Work out the finished part from the listing and answer in its coordinate system (mm). A direction names the side the tool comes from. Round coordinates to 2 decimals unless told otherwise and drop trailing zeros. Write each loop counter-clockwise with the first axis right and the second up, starting at its lowest first coordinate (ties: lowest second). Pieces come first, ordered by that corner, then holes. Notation, with made-up numbers: M 82,74.5 L 126,74.5 A15 ccw 126,93.5 Z; hole C 80,-38 d3. An arc over 180 degrees is marked long. One line per item, written item: value. Start each with the question number.
Q1. Find section C-C (y = 9). Write down the section's boundary in (x, z).
Q2. Find section B-B (z = 3). Write down the section's boundary in (x, y).
Q3. Consider probe 1 along Y at (x, z) = (-27, 1.5); probe 2 along X at (y, z) = (3.5, 1.5); probe 3 along Z at (x, y) = (-9.5, -13). Determine where each line is inside the solid, lowest interval first.
Q4. Given pin 1 Ø1 at (y, z) = (-20.5, 2.5) entering from -X; pin 2 Ø2 at (y, z) = (-31, 2.5) entering from -X; pin 3 Ø1 at (x, z) = (-12.5, 1) entering from +Y, each flat-ended and moving along its own axis, determine where each tip first touches the part or whether it passes through.
Q5. A tool of negligible diameter and unlimited length cuts with its end or side. For faces 4 (the cylindrical face through (4.336, -19.524, 2.465)), 5 (the cylindrical face through (-6.335, 4.375, 6.972)), from which of +Z, -Z, +X, -X, +Y, -Y can it reach the whole face along a straight path? Write none if from no direction.
Q6. Find section A-A (y = 0). Write down the section's boundary in (x, z).
Q7. Find section D-D (z = 7.75). Count the separate pieces of the cut face and the enclosed holes in it, and give its area (3 significant figures).
Q8. The mould has two halves that part along X. Classify faces 1 (the cylindrical face through (-29.11, 26.7, 4.44)), 2 (the flat face through (8, 1, 9)), 3 (the flat face through (-4, 0, 5)): released by +X, released by -X, zero draft, split by the parting line, or undercut.
from build123d import *

# Parameters (mm, degrees)
SKETCH_1_R          = 39.5
EXTRUDE_1_DEPTH     = 9
SKETCH_2_R          = 20
CUT_EXTRUDE_1_DEPTH = 5
SKETCH_3_R          = 1.5
CUT_EXTRUDE_2_DEPTH = 57.581799194
SKETCH_4_R          = 1.5
CUT_EXTRUDE_3_DEPTH = 57.084757288


with BuildPart() as part:
    # 草图1 → 凸台-拉伸1 (new body)
    with BuildSketch(Plane.XY):
        Circle(SKETCH_1_R)
    extrude(amount=EXTRUDE_1_DEPTH)

    # 草图2 → 切除-拉伸1 (cut)
    with BuildSketch(Plane(origin=(0, 0, 0), x_dir=(-1, 0, 0), z_dir=(0, 0, -1))):
        Circle(SKETCH_2_R)
    extrude(amount=-CUT_EXTRUDE_1_DEPTH, mode=Mode.SUBTRACT)

    # 草图3 → 切除-拉伸2 (cut, through all)
    with BuildSketch(Plane(origin=(0, 0, 0), x_dir=(-1, 0, 0), z_dir=(0, 0, -1))):
        with Locations((1.136716128, -32.98041656)):
            Circle(SKETCH_3_R)
        with Locations((-29.130236632, 15.505783236)):
            Circle(SKETCH_3_R)
        with Locations((27.993520504, 17.474633324)):
            Circle(SKETCH_3_R)
    extrude(amount=-CUT_EXTRUDE_2_DEPTH, mode=Mode.SUBTRACT)

    # 草图4 → 切除-拉伸3 (cut, through all)
    with BuildSketch(Plane(origin=(0, 0, 5), x_dir=(-1, 0, 0), z_dir=(0, 0, -1))):
        Circle(SKETCH_4_R)
        with Locations((-4.949747468, 4.949747468)):
            Circle(SKETCH_4_R)
        with Locations((4.949747468, 4.949747468)):
            Circle(SKETCH_4_R)
        with Locations((4.949747468, -4.949747468)):
            Circle(SKETCH_4_R)
        with Locations((-4.949747468, -4.949747468)):
            Circle(SKETCH_4_R)
    extrude(amount=-CUT_EXTRUDE_3_DEPTH, mode=Mode.SUBTRACT)


solid = part.part
The answers:
1. outline: M -38.46,0 L -17.86,0 L -17.86,5 L 17.86,5 L 17.86,0 L 38.46,0 L 38.46,9 L -38.46,9 Z
2. outline: C 0,0 d79; hole C -27.99,17.47 d3; hole C 0,0 d40; hole C -1.14,-32.98 d3; hole C 29.13,15.51 d3
3. probe 1: -28.83 to 16.35, 18.6 to 28.83
3. probe 2: -39.34 to -19.69, 19.69 to 39.34
3. probe 3: 5 to 9
4. pin 1: x = -34.06
4. pin 2: x = -25.7
4. pin 3: y = 37.63
5. face 4: -Z
5. face 5: +Z, -Z
6. outline: M -39.5,0 L -20,0 L -20,5 L -1.5,5 L -1.5,9 L -39.5,9 Z; M 1.5,5 L 20,5 L 20,0 L 39.5,0 L 39.5,9 L 1.5,9 Z
7. separate pieces: 1
7. enclosed holes: 8
7. area: 4,850 mm2
8. face 1: split by the parting line
8. face 2: zero draft
8. face 3: undercut
